Geometry check sheet. Reference: the model listing, model coordinates, mm. A direction names the side the tool comes from. Coordinates: 2 decimals unless noted, no trailing zeros. Write each loop counter-clockwise with the first axis right and the second up, starting at its lowest first coordinate (ties: lowest second). Pieces come first, ordered by that corner, then holes.
from build123d import *

# Parameters (mm, degrees)
F0_W     = 14
F0_H     = 14
F1_DEPTH = 1
F2_W     = 5
F2_H     = 1
F3_DEPTH = 3
F4_R     = 4.99999
F5_DEPTH = 25


# Not quite as in the source:
# - a fillet or chamfer is up to 0.001 mm smaller than in the source, because OpenCascade refuses the exact size


with BuildPart() as f1:
    # F0 (on Top) → F1 (new body)
    with BuildSketch(Plane.XY):
        Rectangle(F0_W, F0_H)
    extrude(amount=F1_DEPTH)

    # F2 (on face) → F3 (join)
    with BuildSketch(Plane.XY.offset(1)):
        Polygon((-1, 1), (-1, 7), (-2, 7), (-2, 2), (-2, 1), align=None)
        with Locations((-4.5, 1.5)):
            Rectangle(F2_W, F2_H)
        Polygon((1, 1), (2, 1), (2, 2), (2, 7), (1, 7), align=None)
        with Locations((4.5, 1.5)):
            Rectangle(F2_W, F2_H)
        with Locations((4.5, -1.5)):
            Rectangle(F2_W, F2_H)
        Polygon((2, -1), (1, -1), (1, -7), (2, -7), (2, -2), align=None)
        with Locations((-4.5, -1.5)):
            Rectangle(F2_W, F2_H)
        Polygon((-2, -7), (-1, -7), (-1, -1), (-2, -1), (-2, -2), align=None)
    extrude(amount=F3_DEPTH)

    # F4 (radius 5 in the source; OpenCascade refuses exactly that, so slightly less here)
    f4_edges = [f1.edges().sort_by_distance(p)[0] for p in [
        (2, -2, 2.5),
        (-1, -1, 2.5),
        (-1, 1, 2.5),
        (1, 1, 2.5),
        (2, 2, 2.5),
        (-2, 2, 2.5),
        (-2, -2, 2.5),
        (1, -1, 2.5),
    ]]
    fillet(f4_edges, radius=F4_R)

    # F5 (cut): faces of the model
    f5_faces = [f1.faces().sort_by_distance(p)[0] for p in [
        (4.8779327776, -4.8779327776, 1),
        (4.8779327776, 4.8779327776, 1),
        (-4.8779327776, 4.8779327776, 1),
        (-4.8779327776, -4.8779327776, 1),
    ]]
    extrude(f5_faces, amount=-F5_DEPTH, mode=Mode.SUBTRACT)


solid = f1.part
1. Sectioned sample at A-A, the plane z = 3.6. Give the number of separate pieces and of enclosed holes in the cut face, and give its area (3 significant figures).
Computed values:
separate pieces: 4
enclosed holes: 0
area: 44.0 mm2
2. Sectioned sample at C-C, the plane y = -4.75. Record the boundary of the cut face in (x, z).
Computed values:
outline: (-2.53, 0) - (2.53, 0) - (2.53, 4) - (1.16, 4) - (1.16, 1) - (-1.16, 1) - (-1.16, 4) - (-2.53, 4) - close
3. Access from +Z, -Z, +X, -X, +Y, -Y to the whole of each face (thin tool, end or side, straight path). Record for faces 1 (the cylindrical face through (3, -4, 2)), 2 (the cylindrical face through (3, -2, 3)), 3 (the flat face through (1, -6.5, 2.5)), 4 (the flat face through (-3, 3, 4)), 5 (the flat face through (6.5, 1, 2.5)).
Computed values:
face 1: +Z, -Z, +X, -Y
face 2: +Z
face 3: +Z, +Y, -Y
face 4: +Z, +X, -X, +Y, -Y
face 5: +Z, +X, -X
4. Draft check along X on faces 6 (the flat face through (-6.5, -1, 2.5)), 7 (the flat face through (0, 1, 1)), 8 (the flat face through (7, 0, 0.6)). Enter one of: released by +X, released by -X, zero draft, split by the parting line, or undercut.
Computed values:
face 6: zero draft
face 7: undercut
face 8: released by +X
5. Gauge pin test, flat ends, axial feed: pin 1 Ø0.5 at (x, z) = (6.5, 3) entering from -Y; pin 2 Ø1.1 at (x, z) = (-6.5, 2.5) entering from +Y; pin 3 Ø0.8 at (y, z) = (6.5, 2) entering from -X. Record the tip position at first contact, or that the pin passes through.
Computed values:
pin 1: stops at y = -2.06
pin 2: stops at y = 2.11
pin 3: stops at x = -2.08
6. Thickness scan on line 1 along Z through (x, y) = (0.25, 3.5); line 2 along Y through (x, z) = (-2.5, 1.05); line 3 along X through (y, z) = (-4.75, 3.5). Record the ranges inside material, lowest first.
Computed values:
line 1: z = 0 to 1
line 2: y = -4.82 to -2.43, 2.43 to 4.82
line 3: x = -2.53 to -1.16, 1.16 to 2.53
